```python
from build123d import *

# Parameters (mm, degrees)
PAD_DEPTH       = 60
SKETCH001_W     = 10
SKETCH001_H     = 7.5
PAD001_DEPTH    = 10
SKETCH002_R     = 2.55
POCKET_DEPTH    = 60
FILLET_R        = 4.99
FILLET001_R     = 1
SKETCH003_R     = 1.4
POCKET001_DEPTH = 7


with BuildPart() as part:
    # Sketch → Pad (new body)
    with BuildSketch(Plane.YZ):
        with BuildLine():
            Line((0, 0), (30, 0))
            Line((30, 0), (30, 3))
            Line((30, 3), (14, 3))
            Line((14, 3), (7.9378221735, 6.5))
            Line((6.205771366, 3.5), (7.9378221735, 6.5))
            ThreePointArc((5.3397459622, 3), (5.8397459622, 3.1339745962), (6.205771366, 3.5))
            Line((0, 3), (5.3397459622, 3))
            Line((0, 0), (0, 3))
        make_face()
    extrude(amount=PAD_DEPTH)

    # Sketch001 (on Face3 of Pad) → Pad001 (join)
    with BuildSketch(Plane(origin=(0, 0, 3), x_dir=(0, -1, 0), z_dir=(0, 0, 1))):
        with Locations((-25, 3.75)):
            Rectangle(SKETCH001_W, SKETCH001_H)
        with Locations((-25, 56.25)):
            Rectangle(SKETCH001_W, SKETCH001_H)
    extrude(amount=PAD001_DEPTH)

    # Sketch002 (on Face15 of Pad001) → Pocket (cut)
    with BuildSketch(Plane(origin=(0, 0, 0), x_dir=(0, 1, 0), z_dir=(-1, 0, 0))):
        with Locations((25, -8)):
            Circle(SKETCH002_R)
    extrude(amount=-POCKET_DEPTH, mode=Mode.SUBTRACT)

    # Fillet
    fillet_edges = [part.edges().sort_by_distance(p)[0] for p in [
        (56.25, 30, 13),
        (56.25, 20, 13),
        (3.75, 30, 13),
        (3.75, 20, 13),
    ]]
    fillet(fillet_edges, radius=FILLET_R)

    # Fillet001
    fillet001_edges = [part.edges().sort_by_distance(p)[0] for p in [
        (7.5, 30, 5.505),
        (0, 30, 4.005),
        (52.5, 30, 5.505),
        (60, 30, 4.005),
        (30, 30, 3),
        (30, 30, 0),
        (60, 15, 0),
        (60, 17, 3),
        (0, 17, 3),
        (0, 15, 0),
        (30, 0, 3),
        (60, 2.669873, 3),
        (0, 2.669873, 3),
        (30, 0, 0),
        (0, 0, 1.5),
        (60, 0, 1.5),
        (52.5, 25, 3),
        (7.5, 25, 3),
        (3.75, 20, 3),
        (56.25, 20, 3),
    ]]
    fillet(fillet001_edges, radius=FILLET001_R)

    # Sketch003 (on Face17 of Fillet) → Pocket001 (cut)
    with BuildSketch(Plane(origin=(0, 4.7990381057, 8.3121778265), x_dir=(0, -0.8660254038, 0.5), z_dir=(0, 0.5, 0.8660254038))):
        with Locations((-7.5, 52)):
            Circle(SKETCH003_R)
        with Locations((-7.5, 8)):
            Circle(SKETCH003_R)
    extrude(amount=-POCKET001_DEPTH, mode=Mode.SUBTRACT)


solid = part.part
```
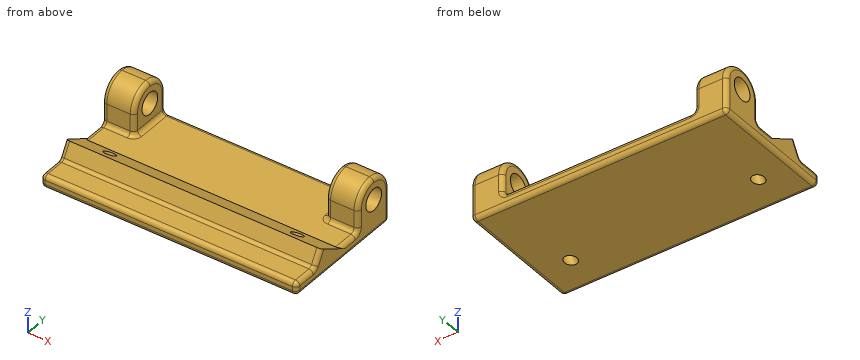
Verification items for the finished model (mm, model axes). Coordinates: 2 decimals unless noted, no trailing zeros. Loops run counter-clockwise (first coordinate to the right, second up) from the corner with the lowest first, then second, coordinate; pieces in that order, holes last. Notation, with made-up numbers: (9.25, 59) -> (25.25, 59) arc R24 cw to (25.25, 94) -> close; hole circle Ø4 at (-9.75, -18.5). An arc over 180 degrees is marked (long way). Answer in a Markdown table with one row per item. Add a question column.
1. Material ranges on probe 1 along Z at (x, y) = (57, 25); probe 2 along Y at (x, z) = (54.75, 8); probe 3 along Z at (x, y) = (51.5, 17), recorded low to high. Write a range as [from, to].
2. Section check B-B, the plane y = 4.5. Enter the section's corners in (x, z).
3. Section check C-C, the plane z = 7.25. Enter the section's corners in (x, y).
4. Section check A-A, the plane x = 14. Enter the section's corners in (y, z), then the cut area to 3 significant figures.
5. Depth check by flat-ended pin: P1, Ø3, axis at x = 56.5, z = 5.5, coming from the -Y side; P2, Ø5, axis at x = 40.5, y = 3.5, coming from the +Z side; P3, Ø5, axis at x = 12.5, y = 6, coming from the +Z side; P4, Ø6, axis at x = 15.5, z = 11, coming from the -Y side. Enter the tip coordinate at first touch or a pass-through.
Derived:
| question | item | result |
|---|---|---|
| 1 | probe 1 | z = [0, 5.45], [10.55, 13] |
| 1 | probe 2 | y = [20, 22.45], [27.55, 30] |
| 1 | probe 3 | z = [0, 3] |
| 2 | outline | (0, 1) arc R1 ccw to (1, 0) -> (59, 0) arc R1 ccw to (60, 1) -> (60, 2) arc R1 ccw to (59, 3) -> (1, 3) arc R1 ccw to (0, 2) -> close |
| 3 | outline | (0, 21) arc R1 ccw to (1, 20) -> (6.5, 20) arc R1 ccw to (7.5, 21) -> (7.5, 22.56) -> (0, 22.56) -> close; (0, 27.44) -> (7.5, 27.44) -> (7.5, 29) arc R1 ccw to (6.5, 30) -> (1, 30) arc R1 ccw to (0, 29) -> close; (52.5, 21) arc R1 ccw to (53.5, 20) -> (59, 20) arc R1 ccw to (60, 21) -> (60, 22.56) -> (52.5, 22.56) -> close; (52.5, 27.44) -> (60, 27.44) -> (60, 29) arc R1 ccw to (59, 30) -> (53.5, 30) arc R1 ccw to (52.5, 29) -> close |
| 4 | outline | (0, 1) arc R1 ccw to (1, 0) -> (29, 0) arc R1 ccw to (30, 1) -> (30, 2) arc R1 ccw to (29, 3) -> (14, 3) -> (7.94, 6.5) -> (6.21, 3.5) arc R1 cw to (5.34, 3) -> (1, 3) arc R1 ccw to (0, 2) -> close |
| 4 | area | 103 mm² |
| 5 | P1 | stops at y = 6.49 |
| 5 | P2 | stops at z = 3.25 |
| 5 | P3 | stops at z = 6.5 |
| 5 | P4 | passes through |
